Autodesk Inventor part; units mm, degrees
ref_plane "YZ Plane" through (0, 0, 0) normal (1, 0, 0) x (0, 1, 0)
ref_plane "XZ Plane" through (0, 0, 0) normal (0, 1, 0) x (-1, 0, 0)
ref_plane "XY Plane" through (0, 0, 0) normal (0, 0, 1) x (1, 0, 0)
sketch "Sketch1" plane through (0, 0, 0) normal (0, 0, 1) x (1, 0, 0)
  line L0 (-9.2684, -9.4429) -> (15.7316, -9.4429)
  line L1 (15.7316, -9.4429) -> (15.7316, 40.5571)
  arc A0 (15.7316, 40.5571) -> (-9.2684, 40.5571) centre (3.2316, 40.5571) ccw
  line L2 (-9.2684, 40.5571) -> (-9.2684, -9.4429)
  circle A1 centre (3.2316, 40.5571) radius 4
  circle A2 centre (-3.7684, 40.5571) radius 1.5
  circle A3 centre (3.2316, 47.5571) radius 1.5
  circle A4 centre (3.2316, 33.5571) radius 1.5
  circle A5 centre (10.2316, 40.5571) radius 1.5
  circle A6 centre (3.2316, 21.9571) radius 1.5
  circle A7 centre (3.2316, 5.0871) radius 1.5
  point P0 (0, 0)
  dimension "d0" = 25
  dimension "d1" = 50
  dimension "d3" = 8
  dimension "d5" = 3
  dimension "d6" = 3
  dimension "d7" = 3
  dimension "d8" = 3
  dimension "d10" = 3
  dimension "d12" = 3
extrude "Extrusion1" add sketch "Sketch1" along normal blind 54
sketch "Sketch2" plane through (15.7316, -9.4429, 0) normal (1, 0, 0) x (0, 0, -1)
  line L0 (-54, 0) -> (-54, 50)
  line L1 (-54, 0) -> (-53, 0)
  line L2 (-53, 0) -> (-53, 1)
  line L3 (-53, 1) -> (-54, 1)
  line L4 (-54, 1) -> (-54, 0)
  line L5 (0, 0) -> (-1, 0)
  line L6 (-1, 0) -> (-1, 1)
  line L7 (-1, 1) -> (0, 1)
  line L8 (0, 1) -> (0, 0)
  line L9 (-53, 1) -> (-53, 62.5)
  line L10 (-53, 1) -> (-1, 1)
  line L11 (-1, 1) -> (-1, 62.5)
  line L12 (0, 50) -> (0, 50)
  line L13 (0, 50) -> (-54, 50)
  line L14 (-54, 50) -> (-54, 50)
  line L15 (0, 50) -> (-54, 50)
  line L16 (0, 62.5) -> (-54, 62.5)
  line L17 (-54, 62.5) -> (-54, 50)
  line L18 (0, 62.5) -> (0, 50)
  line L19 (0, 62.5) -> (-1, 62.5)
  line L20 (-1, 62.5) -> (-1, 0)
  line L21 (-1, 0) -> (0, 0)
  line L22 (0, 0) -> (0, 62.5)
  line L23 (-54, 62.5) -> (-53, 62.5)
  line L24 (-53, 62.5) -> (-53, 0)
  line L25 (-53, 0) -> (-54, 0)
  line L26 (-54, 0) -> (-54, 62.5)
  line L27 (-53, 62.5) -> (-1, 62.5)
  line L28 (-1, 62.5) -> (-1, 1)
  line L29 (-1, 1) -> (-53, 1)
  line L30 (-53, 1) -> (-53, 62.5)
  point P0 (0, 9.4429)
  dimension "d15" = 1
  dimension "d16" = 1
  dimension "d17" = 1
  dimension "d18" = 1
extrude "Extrusion2" cut sketch "Sketch2" against normal through all contours L9 L13 L11 L10 | L9 L16 L11 L13
sketch "Sketch3" plane through (15.7316, -8.4429, 53) normal (0, 1, 0) x (1, 0, 0)
  circle A0 centre (-12.5, 26) radius 4
  circle A1 centre (-12.5, 33) radius 1.5
  circle A2 centre (-19.5, 26) radius 1.5
  circle A3 centre (-12.5, 19) radius 1.5
  circle A4 centre (-5.5, 26) radius 1.5
  circle A5 centre (-12.5, 44.6) radius 1.5
  circle A6 centre (-12.5, 7.4) radius 1.5
  point P0 (-15.7316, 53)
  dimension "d23" = 3
  dimension "d26" = 360
  dimension "d29" = 3
extrude "Extrusion3" cut sketch "Sketch3" against normal blind 58
properties part number "modelo 1"
Source: CAD feature listing. Evaluate the final solid. Frame: model axes, mm. A direction names the side the tool comes from. Give positions to 0.01 mm unless a question says otherwise; leave off trailing zeros. Order: outer loops, then holes, each group sorted by start corner. A loop starts at its lowest first (then second) coordinate and runs counter-clockwise, first axis right, second up.
(1) Material intervals for line 1 along X through (y, z) = (-9.1, 27); line 2 along Z through (x, y) = (6.25, 24.5); line 3 along Y through (x, z) = (1.5, 13.5), sorted ascending.
(2) Access query for faces 1 (the face through (6, 22, 53)), 2 (the face through (6, 22, 54)). Directions: +Z, -Z, +X, -X, +Y, -Y. A direction counts if a zero-diameter tool reaches every point of the face in a straight line with its end or side. Return the directions, or none.
(3) Contact query for a flat-ended pin moving along its axis: P1, Ø5, axis at x = 10.23, z = 27, coming from the +Y side. Output: stop coordinate, or through.
(4) Pull-direction query (Z, two-part tool) for faces 3 (the face through (6, 22, 0)), 4 (the face through (2.71, 36.59, 0.49)), 5 (the face through (3, -8.443, 22)); classes: +Z half, -Z half, draft (parallel to the pull), parting line (faces both ways), or undercut.
(5) Section query C-C (x = 10). Return the cut outline in (y, z).
(6) Section query B-B (y = 14). Return the cut outline in (x, z), plus the area to 3 significant figures.
(7) Section query D-D (x = 0). Return the cut outline in (y, z), plus the area to 3 significant figures.
(8) Section query A-A (z = 34). Return the cut outline in (x, y).
Outcome:
1. line 1: x = -9.27 to -5.27, -2.27 to -0.77, 7.23 to 8.73, 11.73 to 15.73
1. line 2: z = 0 to 1, 53 to 54
1. line 3: y = -9.44 to -8.44
2. face 1: +X, -X, +Y
2. face 2: +Z, +X, -X, +Y, -Y
3. P1: stops at y = -8.44
4. face 3: -Z half
4. face 4: draft
4. face 5: undercut
5. outline: (-9.44, 0) - (39.08, 0) - (39.08, 1) - (-8.44, 1) - (-8.44, 25.52) - (-9.44, 25.52) - close; (-9.44, 28.48) - (-8.44, 28.48) - (-8.44, 53) - (39.08, 53) - (39.08, 54) - (-9.44, 54) - close; (42.04, 0) - (51.07, 0) - (51.07, 1) - (42.04, 1) - close; (42.04, 53) - (51.07, 53) - (51.07, 54) - (42.04, 54) - close
6. outline: (-9.27, 0) - (15.73, 0) - (15.73, 1) - (-9.27, 1) - close; (-9.27, 53) - (15.73, 53) - (15.73, 54) - (-9.27, 54) - close
6. area: 50.0 mm2
7. outline: (-9.44, 0) - (38.2, 0) - (38.2, 1) - (-8.44, 1) - (-8.44, 24.64) - (-9.44, 24.64) - close; (-9.44, 29.36) - (-8.44, 29.36) - (-8.44, 53) - (38.2, 53) - (38.2, 54) - (-9.44, 54) - close; (42.91, 0) - (52.63, 0) - (52.63, 1) - (42.91, 1) - close; (42.91, 53) - (52.63, 53) - (52.63, 54) - (42.91, 54) - close
7. area: 162 mm2
8. outline: (-9.27, -9.44) - (1.73, -9.44) - (1.73, -8.44) - (-9.27, -8.44) - close; (4.73, -9.44) - (15.73, -9.44) - (15.73, -8.44) - (4.73, -8.44) - close
